Could you check a few things on this model? Use its own coordinates, in mm. Round coordinates to 2 decimals unless told otherwise and drop trailing zeros. Write each loop counter-clockwise with the first axis right and the second up, starting at its lowest first coordinate (ties: lowest second). Pieces come first, ordered by that corner, then holes. Notation, with made-up numbers: (-16.5, 43) -> (29.5, 43) arc R13 cw to (29.5, 62) -> close; hole circle Ø1 at (11.5, 30). An arc over 180 degrees is marked (long way). Return JSON: item names as keys, results as strings.
from build123d import *

# Parameters (mm, degrees)
F1_DEPTH = 25.4
F4_DEPTH = 15.875


with BuildPart() as f1:
    # F0 (on Front) → F1 (new body)
    with BuildSketch(Plane.XZ):
        with BuildLine():
            Line((1863.8208496928, 32.7376453102), (-63.4041503072, 32.7376453102))
            Line((-63.4041503072, 32.7376453102), (-63.4041503072, -43.4623546898))
            ThreePointArc((-63.4041503072, -43.4623546898), (900.2083496928, 7.3376453102), (1863.8208496928, -43.4623546898))
            Line((1863.8208496928, -43.4623546898), (1863.8208496928, 32.7376453102))
        make_face()
    extrude(amount=F1_DEPTH)


with BuildPart() as f4:
    # F3 (on Front) → F4 (new body)
    with BuildSketch(Plane.XZ):
        with BuildLine():
            Line((1858.7887722611, 30.7600510478), (-68.4362277389, 30.7600510478))
            Line((-68.4362277389, 30.7600510478), (-68.4362277389, -70.8399489522))
            ThreePointArc((-68.4362277389, -70.8399489521), (895.1762722611, -20.0399489521), (1858.7887722611, -70.8399489521))
            Line((1858.7887722611, -70.8399489522), (1858.7887722611, 30.7600510478))
        make_face()
    extrude(amount=F4_DEPTH)


solid = f4.part
1) If I drill on probe 1 along Z at (x, y) = (1575.5, -9.75); probe 2 along Z at (x, y) = (1429, -9.5), over which ranges is the centre line in solid material (lowest first)? Write a range as [from, to].
Return value:
{"probe 1": "[-45.33, 30.76]", "probe 2": "[-35.6, 30.76]"}
2) I want a section at B-B, the plane y = -11.75. Please give me the cut outline in (x, z).
Return value:
{"outline": "(-68.44, -70.84) arc R9164.66 cw to (1858.79, -70.84) -> (1858.79, 30.76) -> (-68.44, 30.76) -> close"}
3) I want a section at C-C, the plane x = 1583. Please give me the cut outline in (y, z) (3 decimals), and give its area (3 significant figures).
Return value:
{"outline": "(-15.875, -45.888) -> (0, -45.888) -> (0, 30.76) -> (-15.875, 30.76) -> close", "area": "1,220 mm²"}
4) Will this pin go through, and if not, where does the flat tip stop? pin 1 Ø1.5 at (x, z) = (908.5, -2.5) entering from +Y.
Return value:
{"pin 1": "y = 0"}
5) Thinking about a two-plate mould opening in X: for faces 1 (the face through (882, -15.875, -8)), 2 (the face through (881.66, -7.83, -20.05)), which applies, pulls with the +X half, pulls with the -X half, needs draft (parallel to the pull), parting line crosses it, or undercut?
Return value:
{"face 1": "needs draft", "face 2": "undercut"}
